```python
from build123d import *

# Parameters (mm, degrees)
F1_DEPTH = 5
F2_D     = 7
F3_SIZE  = 2


with BuildPart() as f1:
    # F0 (on Front) → F1 (new body)
    with BuildSketch(Plane.XZ):
        Polygon((0, 71.5), (0, 0), (40, 0), (40, 14), (70, 14), (70, 30), (146, 30), (146, 14), (176, 14), (176, 0), (216, 0), (216, 71.5), align=None)
    extrude(amount=-F1_DEPTH)

    # F2 (through all)
    with Locations(Plane.XZ):
        with Locations((203, 58.5), (203, 13), (13, 13), (13, 58.5)):
            Hole(F2_D / 2)

    # F3
    f3_edges = [f1.edges().sort_by_distance(p)[0] for p in [
        (216, 2.5, 71.5),
        (216, 2.5, 0),
        (176, 2.5, 0),
        (40, 2.5, 0),
        (0, 2.5, 0),
        (0, 2.5, 71.5),
    ]]
    chamfer(f3_edges, length=F3_SIZE)


solid = f1.part
```
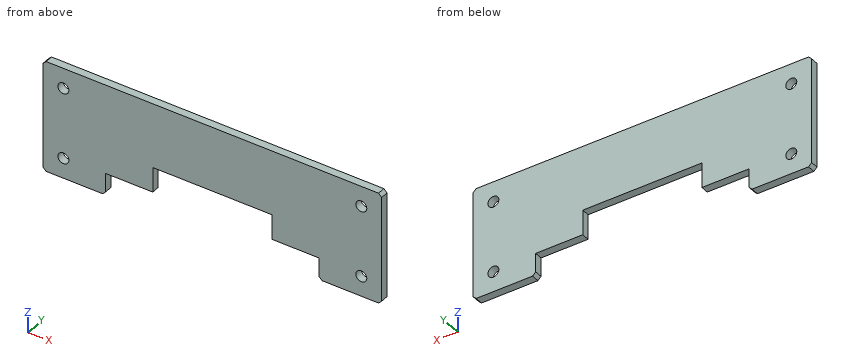
Check sheet for the modelled part. Datum: model origin and axes. Units: mm. Coordinates: 2 decimals unless noted, no trailing zeros. Loops run counter-clockwise (first coordinate to the right, second up) from the corner with the lowest first, then second, coordinate; pieces in that order, holes last.
1) Material ranges on probe 1 along Z at (x, y) = (203, 1.2); probe 2 along X at (y, z) = (3.1, 26.5); probe 3 along X at (y, z) = (0.35, 60.5), recorded low to high.
2) Sectioned sample at D-D (z = 22). Record the boundary of the cut face in (x, y), and give its area (3 significant figures).
3) Sectioned sample at B-B (y = 2.2). Record the boundary of the cut face in (x, z), and give its area (3 significant figures).
4) Sectioned sample at A-A (x = 13). Record the boundary of the cut face in (y, z).
5) Sectioned sample at C-C (z = 58.5). Record the boundary of the cut face in (x, y), and give its area (3 significant figures).
6) Gauge pin test, flat ends, axial feed: pin 1 (2.5 mm diameter, centred on x = 54.5, y = 1.5, fed in from -Z); pin 2 (5.5 mm diameter, centred on x = 203, z = 13, fed in from -Y). Record the tip position at first contact, or that the pin passes through.
Check sheet entries:
1. probe 1: z = 0 to 9.5, 16.5 to 55, 62 to 71.5
1. probe 2: x = 0 to 70, 146 to 216
1. probe 3: x = 0 to 10.13, 15.87 to 200.13, 205.87 to 216
2. outline: (0, 0) - (70, 0) - (70, 5) - (0, 5) - close; (146, 0) - (216, 0) - (216, 5) - (146, 5) - close
2. area: 700 mm2
3. outline: (0, 2) - (2, 0) - (38, 0) - (40, 2) - (40, 14) - (70, 14) - (70, 30) - (146, 30) - (146, 14) - (176, 14) - (176, 2) - (178, 0) - (214, 0) - (216, 2) - (216, 69.5) - (214, 71.5) - (2, 71.5) - (0, 69.5) - close; hole circle Ø7 at (13, 13); hole circle Ø7 at (13, 58.5); hole circle Ø7 at (203, 13); hole circle Ø7 at (203, 58.5)
3. area: 12,200 mm2
4. outline: (0, 0) - (5, 0) - (5, 9.5) - (0, 9.5) - close; (0, 16.5) - (5, 16.5) - (5, 55) - (0, 55) - close; (0, 62) - (5, 62) - (5, 71.5) - (0, 71.5) - close
5. outline: (0, 0) - (9.5, 0) - (9.5, 5) - (0, 5) - close; (16.5, 0) - (199.5, 0) - (199.5, 5) - (16.5, 5) - close; (206.5, 0) - (216, 0) - (216, 5) - (206.5, 5) - close
5. area: 1,010 mm2
6. pin 1: stops at z = 14
6. pin 2: passes through
